Work out the finished part from the listing and answer in its coordinate system (mm). A direction names the side the tool comes from. Coordinates: 2 decimals unless noted, no trailing zeros. Order: outer loops, then holes, each group sorted by start corner. A loop starts at its lowest first (then second) coordinate and runs counter-clockwise, first axis right, second up. Notation, with made-up numbers: (23.5, 20.25) -> (36.5, 20.25) arc R21 ccw to (36.5, 24.25) -> close; hole circle Ø3 at (22.5, -29). An arc over 180 degrees is marked (long way). Answer as CSV lines item,"result". Start each with the question number.
Item 1: Straight lines are drawn through the part: L1, parallel to Y at x = 35, z = 0; L2, parallel to X at y = 110.5, z = -1. For each, find the intervals that lie inside material, in ascending order.
Item 2: For a pull along Y with two mould halves and no side action, classify faces 4 (the face through (34.881, 67.328, 4.614)), 5 (the face through (0, 63, 31.75)), 6 (the face through (-34, 127, -1)) as pulls with the +Y half, pulls with the -Y half, needs draft (parallel to the pull), parting line crosses it, or undercut.
Item 3: Which of the six approach directions +Z, -Z, +X, -X, +Y, -Y give full straight-line access (tool end or side, diameter ignored) to faces 1 (the face through (-34.969, 9.113, 24.796)), 2 (the face through (38.1, 63, 1)), 3 (the face through (0, 63, -31.75))?
Item 4: Section D-D (y = 76.2) is taken. Write down the section's boundary in (x, z), then the cut area to 3 significant figures.
Item 5: Section A-A (z = -18) is taken. Write down the section's boundary in (x, y), then the cut area to 3 significant figures.
Item 6: Each of these flat-tipped pins is pushed along its axis until it touches: pin 1 Ø23 at (y, z) = (34.88, 0.08) entering from +X; pin 2 Ø4 at (y, z) = (11.31, 23.65) entering from -X. Where does it stop, or does it pass through?
Item 7: Section B-B (x = -18.5) is taken. Write down the section's boundary in (y, z), then the cut area to 3 significant figures.
Item 8: Section C-C (y = 89) is taken. Write down the section's boundary in (x, z).
```python
from build123d import *

# Parameters (mm, degrees)
SKETCH1_W           = 76.2
SKETCH1_H           = 76.2
SKETCH1_W_2         = 63.5
SKETCH1_H_2         = 63.5
BOSS_EXTRUDE3_DEPTH = 127
CUT_EXTRUDE4_REACH  = 78.2
SKETCH5_R           = 2.4765
SKETCH5_3_R         = 10
CUT_EXTRUDE5_DEPTH  = 77.2
SKETCH6_R           = 10
CUT_EXTRUDE6_DEPTH  = 77.2


with BuildPart() as part:
    # Sketch1 → Boss-Extrude3 (new body)
    with BuildSketch(Plane(origin=(0, 0, 0), x_dir=(1, 0, 0), z_dir=(0, 1, 0))):
        Rectangle(SKETCH1_W, SKETCH1_H)
        Rectangle(SKETCH1_W_2, SKETCH1_H_2, mode=Mode.SUBTRACT)
    extrude(amount=BOSS_EXTRUDE3_DEPTH)

    # Sketch5 → Cut-Extrude4 (cut, up to next)
    with BuildSketch(Plane.ZY.offset(38.1), mode=Mode.PRIVATE) as cut_extrude4_sk1:
        with Locations((-23.493043794, 58.456697864)):
            Circle(SKETCH5_R)
    cut_extrude4_tool1 = extrude(cut_extrude4_sk1.sketch, amount=-CUT_EXTRUDE4_REACH, mode=Mode.PRIVATE) & part.part
    add(cut_extrude4_tool1.solids().sort_by_distance((-38.1, 58.456698, -23.493044))[0], mode=Mode.SUBTRACT)
    # Sketch5 → Cut-Extrude4 (cut, up to next)
    with BuildSketch(Plane.ZY.offset(38.1), mode=Mode.PRIVATE) as cut_extrude4_sk2:
        with Locations((23.653300841, 58.456697864)):
            Circle(SKETCH5_R)
    cut_extrude4_tool2 = extrude(cut_extrude4_sk2.sketch, amount=-CUT_EXTRUDE4_REACH, mode=Mode.PRIVATE) & part.part
    add(cut_extrude4_tool2.solids().sort_by_distance((-38.1, 58.456698, 23.653301))[0], mode=Mode.SUBTRACT)
    # Sketch5 → Cut-Extrude4 (cut, up to next)
    with BuildSketch(Plane.ZY.offset(38.1), mode=Mode.PRIVATE) as cut_extrude4_sk3:
        with Locations((23.653300841, 11.310353228)):
            Circle(SKETCH5_R)
    cut_extrude4_tool3 = extrude(cut_extrude4_sk3.sketch, amount=-CUT_EXTRUDE4_REACH, mode=Mode.PRIVATE) & part.part
    add(cut_extrude4_tool3.solids().sort_by_distance((-38.1, 11.310353, 23.653301))[0], mode=Mode.SUBTRACT)
    # Sketch5 → Cut-Extrude4 (cut, up to next)
    with BuildSketch(Plane.ZY.offset(38.1), mode=Mode.PRIVATE) as cut_extrude4_sk4:
        with Locations((-23.493043794, 11.310353228)):
            Circle(SKETCH5_R)
    cut_extrude4_tool4 = extrude(cut_extrude4_sk4.sketch, amount=-CUT_EXTRUDE4_REACH, mode=Mode.PRIVATE) & part.part
    add(cut_extrude4_tool4.solids().sort_by_distance((-38.1, 11.310353, -23.493044))[0], mode=Mode.SUBTRACT)

    # Sketch5_3 → Cut-Extrude5 (cut, through all)
    with BuildSketch(Plane.ZY.offset(38.1)):
        with Locations((0.080128523, 34.883525546)):
            Circle(SKETCH5_3_R)
    extrude(amount=-CUT_EXTRUDE5_DEPTH, mode=Mode.SUBTRACT)

    # Sketch6 → Cut-Extrude6 (cut, through all)
    with BuildSketch(Plane.ZY.offset(38.1)):
        with Locations((0, 76.2)):
            Circle(SKETCH6_R)
    extrude(amount=-CUT_EXTRUDE6_DEPTH, mode=Mode.SUBTRACT)


solid = part.part
```
Checked values:
1,L1,"y = 0 to 24.88, 44.88 to 66.2, 86.2 to 127"
1,L2,"x = -38.1 to -31.75, 31.75 to 38.1"
2,face 4,"undercut"
2,face 5,"needs draft"
2,face 6,"pulls with the +Y half"
3,face 1,"-X"
3,face 2,"+Z, -Z, +X, +Y, -Y"
3,face 3,"+Y, -Y"
4,outline,"(-38.1, -38.1) -> (38.1, -38.1) -> (38.1, -10) -> (31.75, -10) -> (31.75, -31.75) -> (-31.75, -31.75) -> (-31.75, -10) -> (-38.1, -10) -> close; (-38.1, 10) -> (-31.75, 10) -> (-31.75, 31.75) -> (31.75, 31.75) -> (31.75, 10) -> (38.1, 10) -> (38.1, 38.1) -> (-38.1, 38.1) -> close"
4,area,"1,520 mm^2"
5,outline,"(-38.1, 0) -> (-31.75, 0) -> (-31.75, 127) -> (-38.1, 127) -> close; (31.75, 0) -> (38.1, 0) -> (38.1, 127) -> (31.75, 127) -> close"
5,area,"1,610 mm^2"
6,pin 1,"stops at x = 38.1"
6,pin 2,"stops at x = 31.75"
7,outline,"(0, -38.1) -> (127, -38.1) -> (127, -31.75) -> (0, -31.75) -> close; (0, 31.75) -> (127, 31.75) -> (127, 38.1) -> (0, 38.1) -> close"
7,area,"1,610 mm^2"
8,outline,"(-38.1, -38.1) -> (38.1, -38.1) -> (38.1, 38.1) -> (-38.1, 38.1) -> close; hole (-31.75, -31.75) -> (31.75, -31.75) -> (31.75, 31.75) -> (-31.75, 31.75) -> close"
